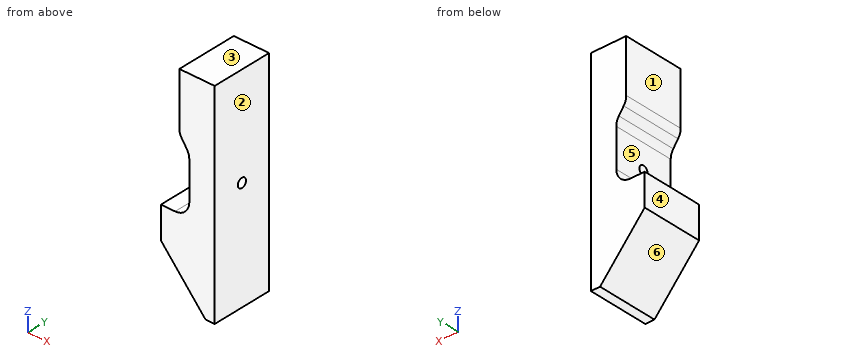
from build123d import *

# Parameters (mm, degrees)
F1_DEPTH = 21.5
F2_R     = 3.25
F3_DEPTH = 17.901
F4_R     = 10


with BuildPart() as f1:
    # F0 (on Front) → F1 (new body, symmetric)
    with BuildSketch(Plane.XZ):
        Polygon((0, -19.4), (-20, -19.4), (-20, -41.812051613), (11.4499329693, -77.827301579), (17.9, -77.827301579), (17.9, 70.8765028308), (-7, 70.8765028308), (-7, 30.6), (0, 20.6), align=None)
    extrude(amount=F1_DEPTH, both=True)

    # F2 (on Right) → F3 (cut, through all)
    with BuildSketch(Plane.YZ):
        Circle(F2_R)
    extrude(amount=F3_DEPTH, mode=Mode.SUBTRACT)

    # F4
    f4_edges = [f1.edges().sort_by_distance(p)[0] for p in [
        (0, 0, -19.4),
        (0, 0, 20.6),
        (-7, 0, 30.6),
    ]]
    fillet(f4_edges, radius=F4_R)


solid = f1.part
CAD build for the part. Positions are in the model's coordinates, mm. Face numbers are marked on the shaded views. A direction names the side the tool comes from. Coordinates: 2 decimals unless noted, no trailing zeros. Order: outer loops, then holes, each group sorted by start corner. A loop starts at its lowest first (then second) coordinate and runs counter-clockwise, first axis right, second up.
Item 1: Band-saw the part on A-A on z = 0. List the corners of the cut face in (x, y).
Check sheet entries:
outline: (0, -21.5) - (17.9, -21.5) - (17.9, -3.25) - (0, -3.25) - close; (0, 3.25) - (17.9, 3.25) - (17.9, 21.5) - (0, 21.5) - close
Item 2: Band-saw the part on B-B on y = 0. List the corners of the cut face in (x, z), plus the area to 3 significant figures.
Check sheet entries:
outline: (-20, -41.81) - (11.45, -77.83) - (17.9, -77.83) - (17.9, -3.25) - (0, -3.25) - (0, -9.4) arc R10 cw to (-10, -19.4) - (-20, -19.4) - close; (-7, 33.75) arc R10 ccw to (-5.19, 28.02) - (-1.81, 23.18) arc R10 cw to (0, 17.45) - (0, 3.25) - (17.9, 3.25) - (17.9, 70.88) - (-7, 70.88) - close
area: 3,490 mm2
Item 3: 3-axis set-ups, long thin cutter, end or side, ignore diameter. For the marked faces 1 and 2: which of +Z, -Z, +X, -X, +Y, -Y reach the whole face in a straight line?
Check sheet entries:
face 1: +Z, -X, +Y, -Y
face 2: +Z, -Z, +X, +Y, -Y
Item 4: Band-saw the part on C-C on y = 9. List the corners of the cut face in (x, z), plus the area to 3 significant figures.
Check sheet entries:
outline: (-20, -41.81) - (11.45, -77.83) - (17.9, -77.83) - (17.9, 70.88) - (-7, 70.88) - (-7, 33.75) arc R10 ccw to (-5.19, 28.02) - (-1.81, 23.18) arc R10 cw to (0, 17.45) - (0, -9.4) arc R10 cw to (-10, -19.4) - (-20, -19.4) - close
area: 3,600 mm2
Item 5: Drill centre lines: L1, parallel to Y at x = 8, z = 0; L2, parallel to Z at x = 13, y = 0; L3, parallel to X at y = 6, z = 63. Where is each one in solid material? Low to high.
Check sheet entries:
L1: y = -21.5 to -3.25, 3.25 to 21.5
L2: z = -77.83 to -3.25, 3.25 to 70.88
L3: x = -7 to 17.9
Item 6: Two-plate mould, pull along Z, no slides. Class the marked faces 3, 4, 5 and 6: +Z half, -Z half, draft (parallel to the pull), parting line (faces both ways), or undercut.
Check sheet entries:
face 3: +Z half
face 4: draft
face 5: undercut
face 6: -Z half
Item 7: Band-saw the part on D-D on z = -69. List the corners of the cut face in (x, y), plus the area to 3 significant figures.
Check sheet entries:
outline: (3.74, -21.5) - (17.9, -21.5) - (17.9, 21.5) - (3.74, 21.5) - close
area: 609 mm2
Item 8: Pin check, flat tips, straight feed: pin 1 Ø13.5 at (y, z) = (-6, 2) entering from -X; pin 2 Ø5 at (y, z) = (-14, -60.5) entering from -X; pin 3 Ø5 at (x, y) = (-17, -10.5) entering from +Z. Stop position of each tip, or through.
Check sheet entries:
pin 1: stops at x = 0
pin 2: stops at x = -5.86
pin 3: stops at z = -19.4
